Verification items for this drawing (mm, ordinates from the low corner). A direction names the side the tool comes from. Coordinates: 2 decimals unless noted, no trailing zeros. Write each loop counter-clockwise with the first axis right and the second up, starting at its lowest first coordinate (ties: lowest second). Pieces come first, ordered by that corner, then holes. Notation, with made-up numbers: M 42,-34.5 L 75,-34.5 A21 cw 75,-14.5 Z; hole C 11,-9.5 d5. An arc over 180 degrees is marked long. Put each result on its own line as item: value. Start each with the question number.
1) Cross-section at B-B on x = 1.1. Record the cut outline in (y, z) (1 decimal).
2) Cross-section at C-C on y = 18. Record the cut outline in (x, z) (1 decimal), plus the area to 3 significant figures.
3) Set-up check for the marked faces 1, 2 and 3: record each of +Z, -Z, +X, -X, +Y, -Y from which the full face is reachable in a straight line by a thin tool's end or side.
4) Gauge pin test, flat ends, axial feed: pin 1 (1.5 mm diameter, centred on x = 3.5, y = 8.5, fed in from +Z); pin 2 (1 mm diameter, centred on x = 0.5, z = 4, fed in from +Y); pin 3 (1 mm diameter, centred on y = 7.5, z = 4, fed in from +X). Record the tip position at first contact, or that the pin passes through.
5) Scan lines: line 1 along Y through (x, z) = (1.75, 0.85); line 2 along Z through (x, y) = (3.4, 6.25) (1 decimal); line 3 along Z through (x, y) = (3.6, 2) (1 decimal). Record each from-to range of solid material in increasing order.
6) Cross-section at A-A on z = 3.65. Record the cut outline in (x, y), plus the area to 3 significant figures.
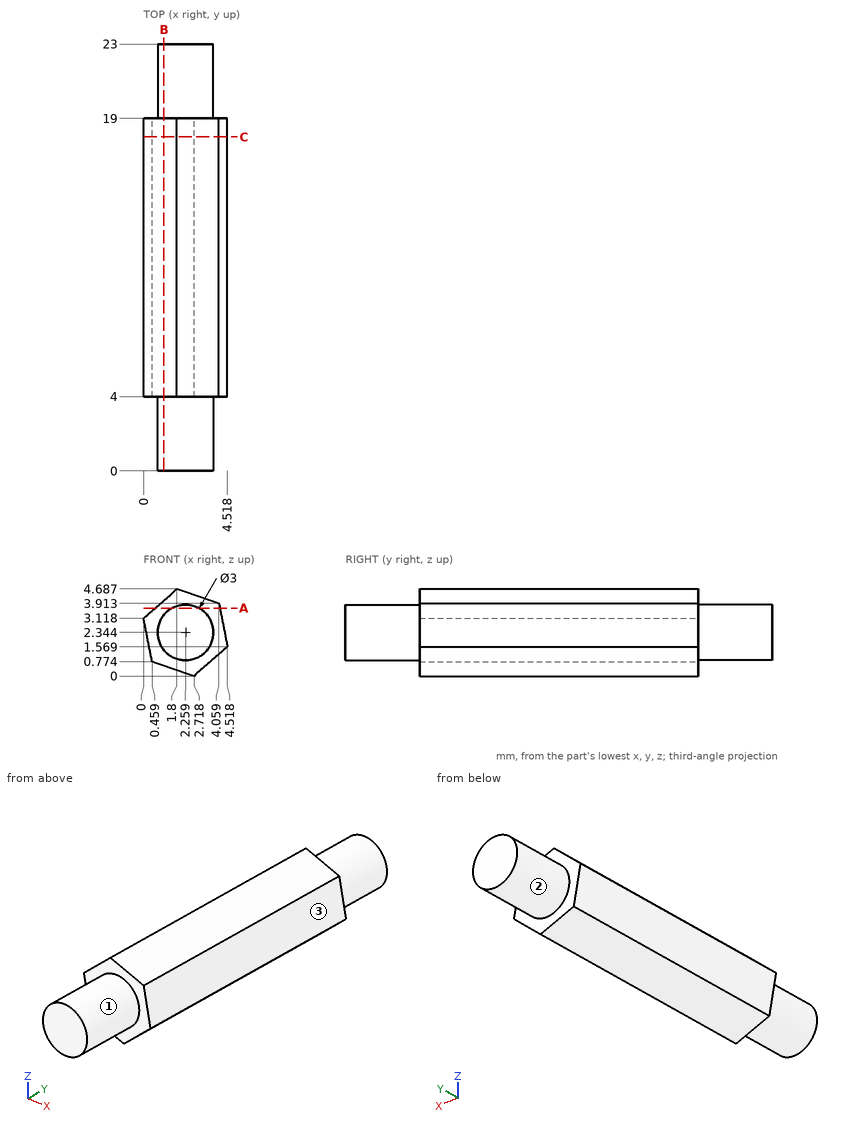
Answer key:
1. outline: M 0,1.4 L 4,1.4 L 4,0.6 L 19,0.6 L 19,1.4 L 23,1.4 L 23,3.3 L 19,3.3 L 19,4.1 L 4,4.1 L 4,3.3 L 0,3.3 Z
2. outline: M 0,3.1 L 0.5,0.8 L 2.7,0 L 4.5,1.6 L 4.1,3.9 L 1.8,4.7 Z
2. area: 14.8 mm²
3. face 1: -Y
3. face 2: +Y
3. face 3: +Z, +X, +Y, -Y
4. pin 1: stops at z = 4.36
4. pin 2: stops at y = 19
4. pin 3: stops at x = 4.14
5. line 1: y = 4 to 19
5. line 2: z = 0.6 to 4.1
5. line 3: z = 1.7 to 3
6. outline: M 0.61,4 L 1.52,4 L 1.52,0 L 3,0 L 3,4 L 4.11,4 L 4.11,19 L 3,19 L 3,23 L 1.52,23 L 1.52,19 L 0.61,19 Z
6. area: 64.3 mm²
